Solid Edge part; units mm, degrees
sketch "Sketch1" plane through (0, 0, 0) normal (0, 0, 1) x (1, 0, 0)
  line L0 (1.5, 0) -> (1.5, 12)
  line L1 (0, 12) -> (1.5, 12)
  line L2 (0, 0) -> (0, 12)
  line L3 (0, 0) -> (0, -3)
  line L4 (0, -3) -> (2.75, -3)
  line L5 (2.75, -3) -> (2.75, 0)
  line L6 (2.75, 0) -> (1.5, 0)
revolve "RevolvedProtrusion1" add sketch "Sketch1" angle 360 about axis through (0, 0, 0) along (0, 1, 0)
sketch "Sketch2" plane through (0, 0, 0) normal (1, 0, 0) x (0, 1, 0)
  line L0 (-3, 1.9365) -> (-1.7, 1.9365)
  line L1 (-0.582, 0) -> (-1.7, 1.9365)
  line L2 (-3, 0) -> (-0.582, 0)
  line L3 (-3, 0) -> (-3, 1.9365)
revolve "RevolvedCutout1" cut sketch "Sketch2" angle 360 about axis through (0, -4.5, 0) along (0, 1, 0)
sketch "Sketch3" plane through (0, -3, 0) normal (0, -1, 0) x (0, 0, 1)
  circle A0 centre (0, 0) radius 1.9365
  line L0 (-1.25, -0.7217) -> (0, -1.4434)
  line L1 (0, -1.4434) -> (1.25, -0.7217)
  line L2 (1.25, -0.7217) -> (1.25, 0.7217)
  line L3 (1.25, 0.7217) -> (0, 1.4434)
  line L4 (0, 1.4434) -> (-1.25, 0.7217)
  line L5 (-1.25, 0.7217) -> (-1.25, -0.7217)
extrude "Protrusion1" add sketch "Sketch3" against normal up to next
sketch "Sketch4" plane through (0, 0, 0) normal (0, 0, 1) x (1, 0, 0)
  line L0 (-1.4434, -3) -> (0, -3)
  line L1 (0, -3) -> (0, -2.6132)
  line L2 (0, -2.6132) -> (-1.4434, -3)
revolve "RevolvedCutout2" cut sketch "Sketch4" angle 360 about axis through (0, -4.5, 0) along (0, 1, 0)
fillet "Round1" radius 0.1 1 edges at (0, 0, -1.5)
fillet "Round2" radius 0.275 1 edges at (0, -3, -2.75)
chamfer "倒斜角_2" distance 0.2 angle 45 1 edges at (0, 12, -1.5)
cosmetic_thread "螺纹_3" thread depth 9.6
Geometry check sheet. Reference: the model listing, model coordinates, mm. A direction names the side the tool comes from. Give positions to 0.01 mm unless a question says otherwise; leave off trailing zeros. Write each loop counter-clockwise with the first axis right and the second up, starting at its lowest first coordinate (ties: lowest second). Pieces come first, ordered by that corner, then holes.
1) Material ranges on L1, parallel to Y at x = -1.6, z = 0.9; L2, parallel to Z at x = -0.8, y = -2; L3, parallel to Z at x = 0.3, y = -1, recorded low to high.
2) Access from +Z, -Z, +X, -X, +Y, -Y to the whole of each face (thin tool, end or side, straight path). Record for faces 1 (the flat face through (-1.08, -2.16, 0.63)), 2 (the cylindrical face through (-1.5, 6.03, -0.07)), 3 (the flat face through (0, 12, 0)).
3) Release check for a two-part mould opening along X. For faces 4 (the flat face through (1.08, -2.16, -0.63)), 5 (the cylindrical face through (-0.596, -1.343, 2.685)), 6 (the flat face through (2, 0, 0)) record: pulls with the +X half, pulls with the -X half, needs draft (parallel to the pull), parting line crosses it, or undercut.
4) Section check A-A, the plane y = 8. Record the boundary of the cut face in (x, z).
5) Gauge pin test, flat end, axial feed: pin 1 (3 mm diameter, centred on x = -2, y = 5, fed in from -Z). Record the tip position at first contact, or that the pin passes through.
Computed:
1. L1: y = -3 to 0
1. L2: z = -2.63 to -1.11, 1.11 to 2.63
1. L3: z = -2.73 to -0.66, 0.66 to 2.73
2. face 1: -Y
2. face 2: +Y
2. face 3: +Z, -Z, +X, -X, +Y
3. face 4: undercut
3. face 5: parting line crosses it
3. face 6: needs draft
4. outline: circle Ø3 at (0, 0)
5. pin 1: stops at z = -1.41
